Autodesk Inventor part; units mm, degrees
ref_plane "YZ Plane" through (0, 0, 0) normal (1, 0, 0) x (0, 1, 0)
ref_plane "XZ Plane" through (0, 0, 0) normal (0, 1, 0) x (-1, 0, 0)
ref_plane "XY Plane" through (0, 0, 0) normal (0, 0, 1) x (1, 0, 0)
sketch "Эскиз1" plane through (0, 0, 0) normal (0, 1, 0) x (-1, 0, 0)
  circle A0 centre (0, 0) radius 3.5
  circle A1 centre (3.5, 0) radius 0.95
  circle A2 centre (-1.75, 3.0311) radius 0.95
  circle A3 centre (-1.75, -3.0311) radius 0.95
  circle A4 centre (0, 0) radius 4.5
  circle A5 centre (0, 0) radius 1.5
  point P0 (-2.5006, -2.4488)
  point P1 (-2.5006, 2.4488)
  point P2 (-0.8704, 3.39)
  point P3 (3.3711, 0.9412)
  point P4 (3.3711, -0.9412)
  point P5 (-0.8704, -3.39)
  dimension "d0" = 7
  dimension "d1" = 1.9
  dimension "d4" = 360
  dimension "d6" = 9
  dimension "d7" = 3
extrude "Выдавливание1" add sketch "Эскиз1" along normal blind 1 contours A0 A1 | A0 A1 | A2 A0 | A0 A2 | A3 A0 | A0 A3 | A4
sketch "Эскиз2" plane through (0, 0, 0) normal (0, -1, 0) x (1, 0, 0)
  circle A0 centre (0, 0) radius 1.5
  circle A1 centre (0, 0) radius 6
  dimension "d10" = 3
  dimension "d11" = 12
extrude "Выдавливание2" add sketch "Эскиз2" along normal blind 5
sketch "Эскиз3" plane through (0, 0, 0) normal (0, 1, 0) x (1, 0, 0)
  circle A0 centre (0, 0) radius 4.5
  circle A1 centre (0, 0) radius 6
  circle A2 centre (0, 0) radius 4.5
  dimension "d14" = 12
extrude "Выдавливание3" add sketch "Эскиз3" along normal blind 5
sketch "Эскиз4" plane through (0, 5, 0) normal (0, 1, 0) x (1, 0, 0)
  arc A0 (0.8704, 3.39) -> (2.5006, 2.4488) centre (1.75, 3.0311) ccw
  line L0 (0, 0) -> (1.75, 3.0311)
  line L1 (0, 0) -> (-5.8023, -10.0499)
  line L2 (-3.2807, -7.6668) -> (-1.0566, -3.645)
  line L3 (-1.0566, -3.645) -> (-2.7193, -2.7255)
  line L4 (-2.7193, -2.7255) -> (-4.9434, -6.7473)
  line L5 (-4.9434, -6.7473) -> (-3.2807, -7.6668)
  circle A1 centre (0, 0) radius 6
  line L6 (-3.2807, -7.6668) -> (-2.7193, -2.7255) construction
  line L7 (-1.0566, -3.645) -> (-4.9434, -6.7473) construction
  point P0 (-3, -5.1962)
  point P1 (-2.1406, -5.6052)
  point P2 (-3.7861, -4.6546)
  dimension "d17" = 1.9
extrude "Выдавливание4" add sketch "Эскиз4" against normal blind 5 contours L3 L2 A1 L1 | L1 A1 L4 L3
sketch "Эскиз5" plane through (0, 5, 0) normal (0, 1, 0) x (1, 0, 0)
  circle A0 centre (0, 0) radius 11.5
  circle A1 centre (0, 0) radius 6
  dimension "d20" = 23
extrude "Выдавливание5" add sketch "Эскиз5" against normal blind 3
properties part number "крышка для втулки"
Input: part model. Units: mm. Frame: model coordinates. A direction names the side the tool comes from. Round coordinates to 2 decimals unless told otherwise and drop trailing zeros. Order: outer loops, then holes, each group sorted by start corner. A loop starts at its lowest first (then second) coordinate and runs counter-clockwise, first axis right, second up. Notation, with made-up numbers: (7.5, 66.25) - (38.5, 66.25) arc R13 cw to (38.5, 81.25) - close; hole circle Ø11 at (80, 59.5). An arc over 180 degrees is marked (long way). Answer as a JSON object with one key per item and string values. Group by question number.
(1) Cut plane B-B (x = 0). Return loops of the section in (y, z), then the cut area to 3 significant figures.
(2) Cut plane D-D (z = -5.25). Return loops of the section in (x, y).
(3) Draft query along X for faces 1 (the face through (3.5, 0.5, 0)), 2 (the face through (-6, -2, 0)), 3 (the face through (5, 5, 0)). Return one class per face: released by +X, released by -X, zero draft, split by the parting line, or undercut.
(4) Cut plane A-A (z = 0). Return loops of the section in (x, y), then the cut area to 4 significant figures.
(5) Cut plane C-C (y = 1.5). Return loops of the section in (x, z) (1 decimal).
(6) Material intervals for probe 1 along Z at (x, y) = (0, -4); probe 2 along Z at (x, y) = (0, 2.35), sorted ascending. Write a range as from..to.
(7) Pin query (flat end, axial travel): P1, Ø1.5, axis at x = -7, z = 6, coming from the -Y side; P2, Ø5, axis at y = 3, z = -6, coming from the -X side; P3, Ø2, axis at x = -1, z = 1.5, coming from the +Y side; P4, Ø2.5, axis at x = 0, z = 0, coming from the -Y side. Return the tip coordinate at first contact, or that it passes through.
(8) Reachability of faces 4 (the face through (-1.88, 3.03, 3.19)), 5 (the face through (-1.5, -2.46, -0.07)), 6 (the face through (5, 2, 5)) from +Z, -Z, +X, -X, +Y, -Y: full face, straight path, thin tool, end or side. Return the list, or none.
Here are the results:
{
 "1": {"outline": "(-5, -6) - (2, -6) - (2, -11.5) - (5, -11.5) - (5, -4.5) - (1, -4.5) - (1, -3.5) - (0, -3.5) - (0, -1.5) - (-5, -1.5) - close; (-5, 1.5) - (0, 1.5) - (0, 3.5) - (1, 3.5) - (1, 4.5) - (5, 4.5) - (5, 11.5) - (2, 11.5) - (2, 6) - (-5, 6) - close", "area": "95.0 mm^2"},
 "2": {"outline": "(-10.23, 2) - (-2.9, 2) - (-2.9, -5) - (2.9, -5) - (2.9, 2) - (10.23, 2) - (10.23, 5) - (-10.23, 5) - close"},
 "3": {"face 1": "undercut", "face 2": "split by the parting line", "face 3": "zero draft"},
 "4": {"outline": "(-11.5, 2) - (-6, 2) - (-6, -5) - (-1.5, -5) - (-1.5, 0) - (-2.55, 0) - (-2.55, 1) - (-4.5, 1) - (-4.5, 5) - (-11.5, 5) - close; (1.5, -5) - (6, -5) - (6, 2) - (11.5, 2) - (11.5, 5) - (4.5, 5) - (4.5, 1) - (3.5, 1) - (3.5, 0) - (1.5, 0) - close", "area": "95.95 mm^2"},
 "5": {"outline": "circle Ø12 at (0, 0); hole (-3, 3.3) arc R4.5 ccw (long way) to (-1.4, 4.3) - (-1.1, 3.6) - (-2.7, 2.7) - close"},
 "6": {"probe 1": "z = -6..-1.5, 1.5..6", "probe 2": "z = -11.5..-4.5, 4.5..11.5"},
 "7": {"P1": "stops at y = 2", "P2": "stops at x = -10.95", "P3": "stops at y = 0", "P4": "passes through"},
 "8": {"face 4": "+Y", "face 5": "+Y, -Y", "face 6": "-Y"}
}
